Input: part model. Units: mm. Frame: model coordinates. Round coordinates to 2 decimals unless told otherwise and drop trailing zeros. Order: outer loops, then holes, each group sorted by start corner. A loop starts at its lowest first (then second) coordinate and runs counter-clockwise, first axis right, second up. Notation, with made-up numbers: M 9.25,1 L 54.25,1 A16 cw 54.25,18 Z; hole C 24.5,-5.75 d11. An arc over 180 degrees is marked long. One line per question, with ' | ' between items.
```python
from build123d import *

# Parameters (mm, degrees)
SKETCH_1_W                = 77.2
SKETCH_1_H                = 78
EXTRUDE_1_DEPTH           = 3
CUT_EXTRUDE_1_DEPTH       = 87
CUT_EXTRUDE_1_DEPTH_BACK  = 71
SKETCH_2_R                = 9.75
CUT_EXTRUDE_3_DEPTH       = 150
CUT_EXTRUDE_3_DEPTH_BACK  = 207
SKETCH_3_R                = 2.4
SKETCH_11_W               = 34.361209151
SKETCH_11_H               = 23.148078535
EXTRUDE_4_DEPTH           = 3
CUT_EXTRUDE_10_DEPTH      = 17
CUT_EXTRUDE_10_DEPTH_BACK = 10
SKETCH_13_R               = 12
CHAMFER_4_SIZE            = 6
SKETCH_14_W               = 38.187974991
SKETCH_14_H               = 34.221306214
EXTRUDE_5_DEPTH           = 3
CUT_EXTRUDE_11_DEPTH      = 644
CUT_EXTRUDE_11_DEPTH_BACK = 12256
SKETCH_15_R               = 12.5
EXTRUDE_6_DEPTH           = 1
EXTRUDE_6_DEPTH_BACK      = 3
SKETCH_16_W               = 18.047356328
SKETCH_16_H               = 3.010605737
SKETCH_17_W               = 19.670999845
SKETCH_17_H               = 3.661099776
CUT_EXTRUDE_12_DEPTH      = 1
FILLET_1_R                = 2


with BuildPart() as part:
    # Эскиз1 → Бобышка-Вытянуть1 (new body)
    with BuildSketch(Plane(origin=(0, 0, 0), x_dir=(1, 0, 0), z_dir=(0, 1, 0))):
        with Locations((-119.576362238, 47.549210869)):
            Rectangle(SKETCH_1_W, SKETCH_1_H)
    extrude(amount=EXTRUDE_1_DEPTH)

    # Эскиз2 → Вырез-Вытянуть1 (cut, two sides: drawn at the far end of the back side and taken through both)
    with BuildSketch(Plane(origin=(0, 3, 0), x_dir=(1, 0, 0), z_dir=(0, 1, 0)).offset(-CUT_EXTRUDE_1_DEPTH_BACK)):
        with Locations(Location((-119.576362238, 22.549210869, 0), (0, 0, 270))):
            Circle(SKETCH_2_R)
    extrude(amount=CUT_EXTRUDE_1_DEPTH + CUT_EXTRUDE_1_DEPTH_BACK, mode=Mode.SUBTRACT)

    # Эскиз3 → Вырез-Вытянуть3 (cut, two sides: drawn at the far end of the back side and taken through both)
    with BuildSketch(Plane(origin=(0, 3, 0), x_dir=(1, 0, 0), z_dir=(0, 1, 0)).offset(-CUT_EXTRUDE_3_DEPTH_BACK)):
        with Locations(Location((-143.176362238, 69.855558065, 0), (0, 0, 270))):
            Circle(SKETCH_3_R)
        with Locations(Location((-143.176362238, 62.855558065, 0), (0, 0, 270))):
            Circle(SKETCH_3_R)
        with Locations(Location((-143.176362238, 55.855558065, 0), (0, 0, 270))):
            Circle(SKETCH_3_R)
        with Locations(Location((-143.176362238, 48.855558065, 0), (0, 0, 270))):
            Circle(SKETCH_3_R)
    extrude(amount=CUT_EXTRUDE_3_DEPTH + CUT_EXTRUDE_3_DEPTH_BACK, mode=Mode.SUBTRACT)

    # Эскиз11 → Бобышка-Вытянуть4 (add)
    with BuildSketch(Plane.XZ):
        with Locations((-119.254790978, -23.284724875)):
            Rectangle(SKETCH_11_W, SKETCH_11_H)
    extrude(amount=-EXTRUDE_4_DEPTH)

    # Эскиз13 → Вырез-Вытянуть10 (cut, two sides: drawn at the far end of the back side and taken through both)
    with BuildSketch(Plane(origin=(0, 3, 0), x_dir=(1, 0, 0), z_dir=(0, 1, 0)).offset(-CUT_EXTRUDE_10_DEPTH_BACK)):
        with Locations(Location((-119.676362238, 27.549210869, 0), (0, 0, 270))):
            Circle(SKETCH_13_R)
    extrude(amount=CUT_EXTRUDE_10_DEPTH + CUT_EXTRUDE_10_DEPTH_BACK, mode=Mode.SUBTRACT)

    # Фаска4
    # the kernel refuses this chamfer: 6 mm, written as the material it takes off along each edge
    with BuildSketch(Plane(origin=(-119.676362238, 0, -27.549210869), x_dir=(0, 0, 1), z_dir=(-1, 0, 0))) as chamfer_4_piece_1:
        Polygon((12 + CHAMFER_4_SIZE, 0), (12, CHAMFER_4_SIZE), (12, 0), align=None)
    revolve(axis=Axis((-119.676362238, 0, -27.549210869), (0, 1, 0)), mode=Mode.SUBTRACT)

    # Эскиз14 → Бобышка-Вытянуть5 (add)
    with BuildSketch(Plane(origin=(0, 3, 0), x_dir=(1, 0, 0), z_dir=(0, 1, 0))):
        with Locations((-119.593003147, 28.62902577)):
            Rectangle(SKETCH_14_W, SKETCH_14_H)
    extrude(amount=-EXTRUDE_5_DEPTH)

    # Эскиз15 → Вырез-Вытянуть11 (cut, two sides: drawn at the far end of the back side and taken through both)
    with BuildSketch(Plane(origin=(0, 3, 0), x_dir=(1, 0, 0), z_dir=(0, 1, 0)).offset(-CUT_EXTRUDE_11_DEPTH_BACK)):
        with Locations(Location((-119.676362238, 25.049210869, 0), (0, 0, 90))):
            Circle(SKETCH_15_R)
    extrude(amount=CUT_EXTRUDE_11_DEPTH + CUT_EXTRUDE_11_DEPTH_BACK, mode=Mode.SUBTRACT)

    # Эскиз16 → Бобышка-Вытянуть6 (add, two sides: drawn at the far end of the back side and taken through both)
    with BuildSketch(Plane.XZ.offset(-EXTRUDE_6_DEPTH_BACK)):
        with Locations((-119.464156945, -10.715514892)):
            Rectangle(SKETCH_16_W, SKETCH_16_H)
    extrude(amount=EXTRUDE_6_DEPTH + EXTRUDE_6_DEPTH_BACK)

    # Эскиз17 → Вырез-Вытянуть12 (cut)
    with BuildSketch(Plane(origin=(0, 0, 0), x_dir=(-1, 0, 0), z_dir=(0, -1, 0))):
        with Locations((119.795379251, 10.745864147)):
            Rectangle(SKETCH_17_W, SKETCH_17_H)
    extrude(amount=CUT_EXTRUDE_12_DEPTH, mode=Mode.SUBTRACT)

    # Скругление1
    fillet_1_edges = [part.edges().sort_by_distance(p)[0] for p in [
        (-119.676362238, 0, -12.549210869),
    ]]
    fillet(fillet_1_edges, radius=FILLET_1_R)


solid = part.part
```
Item 1: Section query C-C, the plane z = -63. Return loops of the section in (x, y).
Report:
outline: M -158.18,0 L -145.57,0 L -145.57,3 L -158.18,3 Z; M -140.78,0 L -80.98,0 L -80.98,3 L -140.78,3 Z
Item 2: Section query B-B, the plane y = 0.7. Return loops of the section in (x, z).
Report:
outline: M -158.18,-86.55 L -80.98,-86.55 L -80.98,-8.55 L -158.18,-8.55 Z; hole C -143.18,-69.86 d4.8; hole C -143.18,-62.86 d4.8; hole C -143.18,-55.86 d4.8; hole C -143.18,-48.86 d4.8; hole C -119.68,-25.05 d25.96
Item 3: Mould query, pull axis Z, two halves, no side actions, for faces 1 (the cylindrical face through (-141.15, 1.48, -68.57)), 2 (the cylindrical face through (-140.8, 1.5, -49.2)), 3 (the flat face through (-120, 0, -48)), 4 (the flat face through (-120, 1, -86.549)). Classes: +Z half, -Z half, draft (parallel to the pull), parting line (faces both ways), or undercut.
Report:
face 1: undercut | face 2: undercut | face 3: draft | face 4: -Z half
Item 4: Line query: line 1 along X through (y, z) = (1.2, -23); line 2 along Z through (x, y) = (-141.5, 1.5); line 3 along X through (y, z) = (2.1, -33). Output: solid intervals per line, ascending. Write a range as from..to.
Report:
line 1: -158.18..-132.18, -107.18..-80.98 | line 2: -86.55..-71.57, -68.14..-64.57, -61.14..-57.57, -54.14..-50.57, -47.14..-8.55 | line 3: -158.18..-129.32, -110.03..-80.98
Item 5: Section query A-A, the plane z = -47.5. Return loops of the section in (x, y).
Report:
outline: M -158.18,0 L -145.16,0 L -145.16,3 L -158.18,3 Z; M -141.2,0 L -80.98,0 L -80.98,3 L -141.2,3 Z
